The model under review builds one solid part; all positions refer to its coordinate system, in mm. A direction names the side the tool comes from. Round coordinates to 2 decimals unless told otherwise and drop trailing zeros. Order: outer loops, then holes, each group sorted by start corner. A loop starts at its lowest first (then second) coordinate and runs counter-clockwise, first axis right, second up.
```python
from build123d import *

# Parameters (mm, degrees)
BOSS_EXTRUDE1_DEPTH                                = 11
BOSS_EXTRUDE2_DEPTH                                = 36
BOSS_EXTRUDE3_DEPTH                                = 11
CUT_EXTRUDE1_DEPTH                                 = 19.5
CUT_EXTRUDE2_DEPTH                                 = 19.5
F_3_9_3_9_DIAMETER_HOLE1_D                         = 3.9
F_3_9_3_9_DIAMETER_HOLE1_DEPTH                     = 30
F_3_9_3_9_DIAMETER_HOLE1_TIP                       = 1.171678207
CBORE_FOR_M3_5_HEX_HEAD_MACHINE_SCREW1_D           = 4
CBORE_FOR_M3_5_HEX_HEAD_MACHINE_SCREW1_DEPTH       = 40.80674334
CBORE_FOR_M3_5_HEX_HEAD_MACHINE_SCREW1_CBORE_D     = 12
CBORE_FOR_M3_5_HEX_HEAD_MACHINE_SCREW1_CBORE_DEPTH = 19.5
F_4_0_4_DIAMETER_HOLE1_D                           = 4
F_4_0_4_DIAMETER_HOLE1_DEPTH                       = 21.30674334
CHAMFER1_SIZE                                      = 2
FILLET4_R                                          = 5
FILLET5_R                                          = 6
CUT_EXTRUDE3_DEPTH                                 = 141.586272594


with BuildPart() as part:
    # Sketch1 → Boss-Extrude1 (new body)
    with BuildSketch(Plane(origin=(-29, 0, 0), x_dir=(0, -1, 0), z_dir=(-1, 0, 0))):
        Polygon((125.5, 25.5), (84.69325666, 25.5), (98.358665474, -25.5), (125.5, -25.5), align=None)
    extrude(amount=-BOSS_EXTRUDE1_DEPTH)

    # Sketch2 → Boss-Extrude2 (add)
    with BuildSketch(Plane(origin=(-18, 0, 0), x_dir=(0, 0, -1), z_dir=(1, 0, 0))):
        Polygon((25.5, -107.179491924), (15.5, -104.5), (9.873066959, -125.5), (-25.5, -125.5), (-25.5, -84.69325666), (25.5, -98.358665474), align=None)
    extrude(amount=BOSS_EXTRUDE2_DEPTH)

    # Sketch3 → Boss-Extrude3 (add)
    with BuildSketch(Plane(origin=(18, 0, 0), x_dir=(0, 0, -1), z_dir=(1, 0, 0))):
        Polygon((-25.5, -125.5), (-25.5, -84.69325666), (25.5, -98.358665474), (25.5, -125.5), align=None)
    extrude(amount=BOSS_EXTRUDE3_DEPTH)

    # Sketch4 → Cut-Extrude1 (cut)
    with BuildSketch(Plane.XZ.offset(125.5)):
        with BuildLine():
            Line((29, -25.5), (29, -16.626602828))
            ThreePointArc((29, -16.626602828), (21.350933194, -17.165805191), (20.478555895, -24.784067463))
            Line((20.478555895, -24.784067463), (20.478555895, -25.5))
            Line((20.478555895, -25.5), (29, -25.5))
        make_face()
    extrude(amount=-CUT_EXTRUDE1_DEPTH, mode=Mode.SUBTRACT)

    # Sketch5 → Cut-Extrude2 (cut)
    with BuildSketch(Plane.XZ.offset(125.5)):
        with BuildLine():
            Line((-20.478555895, -25.5), (-20.478555895, -24.784067463))
            ThreePointArc((-20.478555895, -24.784067463), (-21.350933194, -17.165805191), (-29, -16.626602828))
            Line((-29, -16.626602828), (-29, -25.5))
            Line((-29, -25.5), (-20.478555895, -25.5))
        make_face()
    extrude(amount=-CUT_EXTRUDE2_DEPTH, mode=Mode.SUBTRACT)

    # Ø3.9 (3.9) Diameter Hole1
    with Locations(Plane(origin=(0, -10.875172652, -40.586696879), x_dir=(-1, 0, 0), z_dir=(0, -0.25881904510251963, -0.9659258262890685))):
        with Locations((0, -111.918353437), (-11, -111.918353437), (-5.5, -104.418353437), (5.5, -104.418353437), (11, -111.918353437)):
            Hole(F_3_9_3_9_DIAMETER_HOLE1_D / 2, depth=F_3_9_3_9_DIAMETER_HOLE1_DEPTH)
            with Locations((0, 0, -(F_3_9_3_9_DIAMETER_HOLE1_DEPTH + F_3_9_3_9_DIAMETER_HOLE1_TIP / 2))):  # 118° drill point
                Cone(0, F_3_9_3_9_DIAMETER_HOLE1_D / 2, F_3_9_3_9_DIAMETER_HOLE1_TIP, mode=Mode.SUBTRACT)

    # CBORE for M3.5 Hex Head Machine Screw1
    with Locations(Plane(origin=(0, -125.5, 0), x_dir=(-1, 0, 0), z_dir=(0, -1, 0))):
        with Locations((-25.5, -12.5)):
            CounterBoreHole(CBORE_FOR_M3_5_HEX_HEAD_MACHINE_SCREW1_D / 2, CBORE_FOR_M3_5_HEX_HEAD_MACHINE_SCREW1_CBORE_D / 2, CBORE_FOR_M3_5_HEX_HEAD_MACHINE_SCREW1_CBORE_DEPTH, depth=CBORE_FOR_M3_5_HEX_HEAD_MACHINE_SCREW1_DEPTH)

    # Ø4.0 (4) Diameter Hole1
    with Locations(Plane(origin=(0, -106, 0), x_dir=(-1, 0, 0), z_dir=(0, -1, 0))):
        with Locations((25.5, 21.5), (-25.5, 21.5)):
            Hole(F_4_0_4_DIAMETER_HOLE1_D / 2, depth=F_4_0_4_DIAMETER_HOLE1_DEPTH)

    # Chamfer1
    chamfer1_edges = [part.edges().sort_by_distance(p)[0] for p in [
        (29, -105.09662833, 25.5),
        (29, -102.179332737, -25.5),
        (-29, -102.179332737, -25.5),
        (-29, -105.09662833, 25.5),
        (-29, -125.5, 4.436698586),
    ]]
    chamfer(chamfer1_edges, length=CHAMFER1_SIZE)

    # Fillet4
    fillet4_edges = [part.edges().sort_by_distance(p)[0] for p in [
        (19.239277947, -125.5, -25.5),
        (-19.239277947, -125.5, -25.5),
    ]]
    fillet(fillet4_edges, radius=FILLET4_R)

    # Fillet5
    fillet5_edges = [part.edges().sort_by_distance(p)[0] for p in [
        (-18, -105.839745962, -20.5),
        (18, -105.839745962, -20.5),
    ]]
    fillet(fillet5_edges, radius=FILLET5_R)

    # Sketch12 → Cut-Extrude3 (cut, through all)
    with BuildSketch(Plane(origin=(29, 0, 0), x_dir=(0, 0, -1), z_dir=(1, 0, 0))):
        with BuildLine():
            Line((0, -125.5), (-25.5, -125.5))
            Line((-25.5, -125.5), (-25.5, -100))
            ThreePointArc((-25.5, -100), (-18.03122292, -118.03122292), (0, -125.5))
        make_face()
    extrude(amount=-CUT_EXTRUDE3_DEPTH, mode=Mode.SUBTRACT)


solid = part.part
```
(1) Consider section A-A (x = -25.5). Write out the cut boundary in (y, z), and give its area (3 significant figures).
Data:
outline: (-125.5, -15.5) - (-106, -15.5) - (-106, -19.5) - (-96.75, -19.5) - (-84.69, 25.5) - (-100, 25.5) arc R25.5 ccw to (-125.5, 0) - close; (-106, -25.5) - (-98.36, -25.5) - (-97.82, -23.5) - (-106, -23.5) - close
area: 1,360 mm2
(2) Consider section B-B (y = -90.5). Write out the cut boundary in (x, z).
Data:
outline: (-29, 3.83) - (29, 3.83) - (29, 23.5) - (27, 25.5) - (-27, 25.5) - (-29, 23.5) - close; hole circle Ø4 at (25.5, 12.5)
(3) Insertion check: pin 1 (4.5 mm diameter, centred on x = -25.5, z = -21.5, fed in from -Y); pin 2 (0.8 mm diameter, centred on y = -118, z = -25.5, fed in from -X); pin 3 (5 mm diameter, centred on x = -21, z = 10, fed in from -Y). Each pin has a flat end and moves straight along its axis. Give the tip position at first contact, or say it passes through.
Data:
pin 1: stops at y = -106
pin 2: stops at x = -20.48
pin 3: stops at y = -124.37
(4) For faces 1 (the cylindrical face through (21.436, -115.886, -17.086)), 2 (the flat face through (28, -101.9, -24.5)), 3 (the conical face through (5.544, -103.396, 16.265)), list the 3-axis set-ups (+Z, -Z, +X, -X, +Y, -Y) from which the entire face can be reached by the end or side of a thin tool; tool diameter is ignored.
Data:
face 1: -Y
face 2: -Z, +X, +Y, -Y
face 3: none
(5) Consider section D-D (z = 12.5). State how many separate pieces and enclosed holes the cut face has, and give its area (3 significant figures).
Data:
separate pieces: 2
enclosed holes: 5
area: 1,690 mm2
(6) To check wall thickness, follow probe 1 along X at (y, z) = (-109, -3); probe 2 along X at (y, z) = (-103.25, -21.5); probe 3 along Z at (x, y) = (25.5, -103.5). State the ranges of each line that lie inside material, in increasing order.
Data:
probe 1: x = -29 to -7.45, -3.55 to 3.55, 7.45 to 29
probe 2: x = -29 to -27.5, -23.5 to 23.5, 27.5 to 29
probe 3: z = -25.5 to -23.5, -19.5 to 10.5, 14.5 to 25.26
(7) Consider section C-C (x = 25.5). Write out the cut boundary in (y, z).
Data:
outline: (-125.5, -15.5) - (-106, -15.5) - (-106, -19.5) - (-96.75, -19.5) - (-88.71, 10.5) - (-106, 10.5) - (-106, 6.5) - (-124.66, 6.5) arc R25.5 ccw to (-125.5, 0) - close; (-117.55, 18.5) - (-106, 18.5) - (-106, 14.5) - (-87.64, 14.5) - (-84.69, 25.5) - (-100, 25.5) arc R25.5 ccw to start; (-106, -25.5) - (-98.36, -25.5) - (-97.82, -23.5) - (-106, -23.5) - close
(8) Draft analysis for pull direction X (two halves, no side actions). For faces 4 (the cylindrical face through (20.115, -113.386, 9.854)), 5 (the cylindrical face through (4.06, -106.53, 0.79)), 6 (the flat face through (28, -94.7, 24.5)), 7 (the flat face through (-28, -101.9, -24.5)), state which applies: pulls with the +X half, pulls with the -X half, needs draft (parallel to the pull), parting line crosses it, or undercut.
Data:
face 4: undercut
face 5: undercut
face 6: pulls with the +X half
face 7: pulls with the -X half
